Design review of the part shown in the three views and the two pictorial views. Dimensions are in mm from the part's minimum x, y and z. Give positions to 0.01 mm unless a question says otherwise; leave off trailing zeros. Loops run counter-clockwise (first coordinate to the right, second up) from the corner with the lowest first, then second, coordinate; pieces in that order, holes last. Notation, with made-up numbers: M 9,45.25 L 33,45.25 A31 cw 33,81.25 Z; hole C -40,83 d3. An arc over 180 degrees is marked long. Return JSON: item names as keys, results as strings. Group by question number.
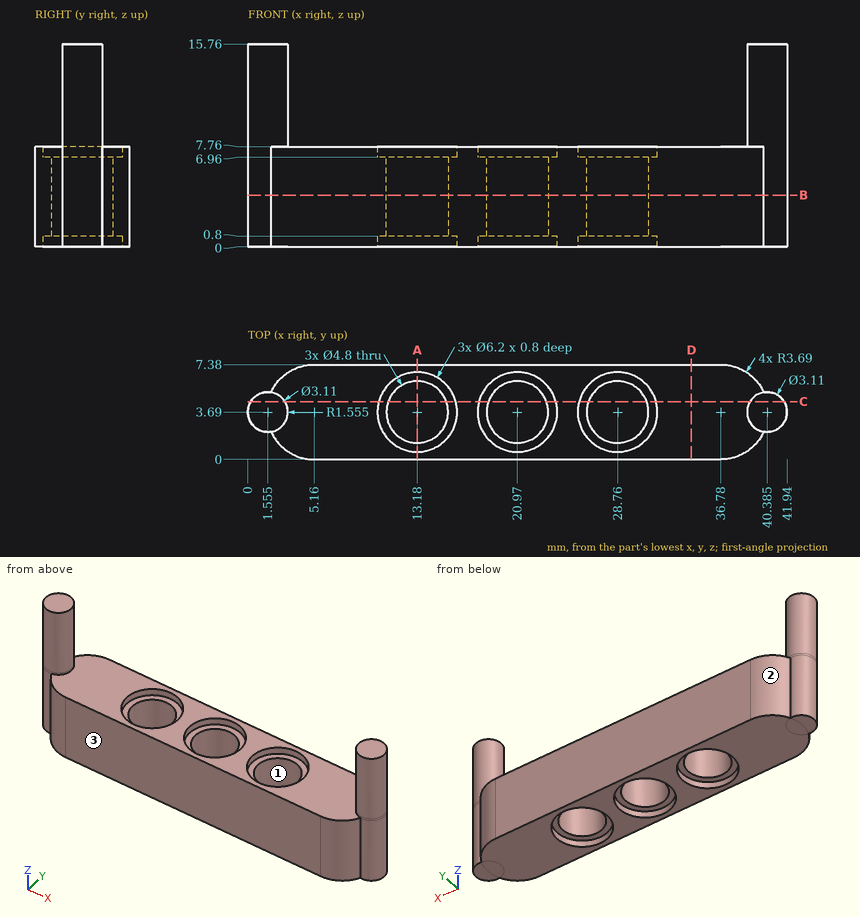
(1) Add section B-B (z = 4). Write out the cut boundary in (x, y) (1 decimal), and give its area (3 significant figures).
(2) For pin 1 (1 mm diameter, centred on x = 31.5, y = 3, fed in from +Z); pin 2 (4 mm diameter, centred on x = 29, z = 7.5, fed in from -Y); pin 3 (1.9 mm diameter, centred on x = 13.5, y = 5, fed in from -Z); pin 4 (1.9 mm diameter, centred on x = 11.5, y = 4.5, fed in from +Z), all flat-tipped, find the tip position at first contact; note any pin that passes through.
(3) For probe 1 along Y at (x, z) = (13.18, 0.4); probe 2 along Y at (x, z) = (20.97, 5.75); probe 3 along Z at (x, y) = (25.5, 5.75), list the stretches that pass through material, from the lowest coordinate up.
(4) Add section A-A (x = 13.18). Write out the cut boundary in (y, z).
(5) Add section C-C (y = 4.5). Count the separate pieces of the cut face and the enclosed holes in it, and give its area (3 significant figures).
(6) Mouldability with a two-part tool opening along Y and no side actions: class the marked faces 1, 2 and 3 as released by +Y, released by -Y, zero draft, split by the parting line, or undercut.
(7) Add section D-D (x = 34.5). Write out the cut boundary in (y, z).
Verdict:
{
 "1": {"outline": "M 1.8,2.2 A3.7 ccw 5.2,0 L 36.8,0 A3.7 ccw 40.1,2.2 A1.6 ccw long 40.1,5.2 A3.7 ccw 36.8,7.4 L 5.2,7.4 A3.7 ccw 1.8,5.2 A1.6 ccw long Z; hole C 13.2,3.7 d4.8; hole C 21,3.7 d4.8; hole C 28.8,3.7 d4.8", "area": "230 mm²"},
 "2": {"pin 1": "stops at z = 7.76", "pin 2": "stops at y = 0", "pin 3": "passes through", "pin 4": "stops at z = 6.96"},
 "3": {"probe 1": "y = 0 to 0.59, 6.79 to 7.38", "probe 2": "y = 0 to 1.29, 6.09 to 7.38", "probe 3": "z = 0 to 7.76"},
 "4": {"outline": "M 0,0 L 0.59,0 L 0.59,0.8 L 1.29,0.8 L 1.29,6.96 L 0.59,6.96 L 0.59,7.76 L 0,7.76 Z; M 6.09,0.8 L 6.79,0.8 L 6.79,0 L 7.38,0 L 7.38,7.76 L 6.79,7.76 L 6.79,6.96 L 6.09,6.96 Z"},
 "5": {"separate pieces": "4", "enclosed holes": "0", "area": "252 mm²"},
 "6": {"face 1": "undercut", "face 2": "released by +Y", "face 3": "released by -Y"},
 "7": {"outline": "M 0,0 L 7.38,0 L 7.38,7.76 L 0,7.76 Z"}
}
